from build123d import *

# Parameters (mm, degrees)
ESQUISSE1_W             = 27.85
ESQUISSE1_H             = 200
BOSS_EXTRU_1_DEPTH      = 6
ESQUISSE4_R             = 2.5
ENL_V_MAT_EXTRU_3_DEPTH = 29
ESQUISSE5_R             = 13.925
ENL_V_MAT_EXTRU_4_DEPTH = 3
ESQUISSE7_W             = 16.87
ESQUISSE7_H             = 23
ESQUISSE7_H_2           = 29
ENL_V_MAT_EXTRU_6_DEPTH = 13
CONG_1_R                = 10
CONG_2_R                = 10


with BuildPart() as part:
    # Esquisse1 → Boss.-Extru.1 (new body)
    with BuildSketch(Plane.XY):
        with Locations((4.111190476, -68.237738095)):
            Rectangle(ESQUISSE1_W, ESQUISSE1_H)
        with BuildLine():
            Line((-9.813809524, 31.762261905), (18.036190476, 31.762261905))
            ThreePointArc((18.036190476, 31.762261905), (4.111190476, 45.687261905), (-9.813809524, 31.762261905))
        make_face()
    extrude(amount=BOSS_EXTRU_1_DEPTH)

    # Esquisse4 → Enlèv. mat.-Extru.3 (cut)
    with BuildSketch(Plane.XY.offset(6)):
        with Locations((4.111190476, -160.237738095)):
            Circle(ESQUISSE4_R)
    extrude(amount=-ENL_V_MAT_EXTRU_3_DEPTH, mode=Mode.SUBTRACT)

    # Esquisse5 → Enlèv. mat.-Extru.4 (cut)
    with BuildSketch(Plane(origin=(0, 0, 0), x_dir=(-1, 0, 0), z_dir=(0, 0, -1))):
        with Locations((-4.111190476, 31.762261905)):
            Circle(ESQUISSE5_R)
    extrude(amount=-ENL_V_MAT_EXTRU_4_DEPTH, mode=Mode.SUBTRACT)

    # Esquisse7 → Enlèv. mat.-Extru.6 (cut)
    with BuildSketch(Plane(origin=(0, 0, 0), x_dir=(-1, 0, 0), z_dir=(0, 0, -1))):
        with BuildLine():
            ThreePointArc((-13.036190476, -115.237738095), (-4.601190476, -106.802738095), (3.833809524, -115.237738095))
            Line((3.833809524, -115.237738095), (-13.036190476, -115.237738095))
        make_face()
        with Locations((-4.601190476, -126.737738095)):
            Rectangle(ESQUISSE7_W, ESQUISSE7_H)
        with BuildLine():
            Line((-13.036190476, -138.237738095), (3.833809524, -138.237738095))
            ThreePointArc((3.833809524, -138.237738095), (-4.601190476, -146.672738095), (-13.036190476, -138.237738095))
        make_face()
        with BuildLine():
            Line((3.833809524, -93.237738095), (-13.036190476, -93.237738095))
            ThreePointArc((-13.036190476, -93.237738095), (-4.601190476, -101.672738095), (3.833809524, -93.237738095))
        make_face()
        with Locations((-4.601190476, -78.737738095)):
            Rectangle(ESQUISSE7_W, ESQUISSE7_H_2)
        with BuildLine():
            Line((3.833809524, -64.237738095), (-13.036190476, -64.237738095))
            ThreePointArc((-13.036190476, -64.237738095), (-4.601190476, -55.802738095), (3.833809524, -64.237738095))
        make_face()
        with BuildLine():
            ThreePointArc((3.833809524, -42.237738095), (-4.601190476, -50.672738095), (-13.036190476, -42.237738095))
            Line((-13.036190476, -42.237738095), (3.833809524, -42.237738095))
        make_face()
        with Locations((-4.601190476, -30.737738095)):
            Rectangle(ESQUISSE7_W, ESQUISSE7_H)
        with BuildLine():
            Line((3.833809524, -19.237738095), (-13.036190476, -19.237738095))
            ThreePointArc((-13.036190476, -19.237738095), (-4.601190476, -10.802738095), (3.833809524, -19.237738095))
        make_face()
    extrude(amount=-ENL_V_MAT_EXTRU_6_DEPTH, mode=Mode.SUBTRACT)

    # Congé1
    cong_1_edges = [part.edges().sort_by_distance(p)[0] for p in [
        (18.036190476, -168.237738095, 3),
    ]]
    fillet(cong_1_edges, radius=CONG_1_R)

    # Congé2
    cong_2_edges = [part.edges().sort_by_distance(p)[0] for p in [
        (-9.813809524, -168.237738095, 3),
    ]]
    fillet(cong_2_edges, radius=CONG_2_R)


solid = part.part
Here's how the part is built. I have some questions about the finished solid (model axes, mm). A direction names the side the tool comes from. Coordinates: 2 decimals unless noted, no trailing zeros. Loops run counter-clockwise (first coordinate to the right, second up) from the corner with the lowest first, then second, coordinate; pieces in that order, holes last. Notation, with made-up numbers: (60, 16.25) -> (87, 16.25) arc R15 ccw to (87, 23.25) -> close; hole circle Ø1 at (12, 54.5). An arc over 180 degrees is marked (long way). Use one line per item in the form item = value. Start each with the question number.
(1) On a 3-axis mill with a long thin cutter (end or side, diameter ignored), from which of +Z, -Z, +X, -X, +Y, -Y can I reach the whole of each face in a straight line? I mean faces 1 (the face through (-6.807, -165.386, 3.042)), 2 (the face through (4.787, -10.805, 2.958)), 3 (the face through (4, 32, 3)). Say none if no direction works.
(2) If we section it at B-B (z = 1.8): Please give me the cut outline in (x, y) (3 decimals), then the cut area to 3 significant figures.
(3) If we section it at A-A (y = -47): Please give me the cut outline in (x, z), then the cut area to 3 significant figures.
(4) If we section it at C-C (y = -142): Please give me the cut outline in (x, z).
(5) We'd pull the mould along X, two halves only. Please class faces 4 (the face through (18.036, -65, 3)), 5 (the face through (3.79, -157.76, 3.04)), 6 (the face through (-9.814, -65, 3)), 7 (the face through (-5, -60, 6)): pulls with the +X half, pulls with the -X half, needs draft (parallel to the pull), parting line crosses it, or undercut.
(6) Will these pins go through, and if not, where does the flat tip stop? pin 1 (3 mm diameter, centred on x = 12, z = 1, fed in from +Y); pin 2 (2 mm diameter, centred on x = 15, z = 5, fed in from +Y).
(7) Please list where these lines run through material, in increasing order: line 1 along Y through (x, z) = (12.25, 4.55); line 2 along X through (y, z) = (-21.5, 0.5); line 3 along Y through (x, z) = (11, 1.85).
Verdict:
q1.face_1 = +Z, -Z, -X, -Y
q1.face_2 = +Z, -Z
q1.face_3 = -Z, +Y
q2.outline = (-9.814, -158.238) arc R10 ccw to (0.186, -168.238) -> (8.036, -168.238) arc R10 ccw to (18.036, -158.238) -> (18.036, 31.762) arc R13.925 cw to (-9.814, 31.762) -> close; hole (-3.834, -138.238) arc R8.435 ccw to (13.036, -138.238) -> (13.036, -115.238) arc R8.435 ccw to (-3.834, -115.238) -> close; hole (-3.834, -93.238) arc R8.435 ccw to (13.036, -93.238) -> (13.036, -64.238) arc R8.435 ccw to (-3.834, -64.238) -> close; hole (-3.834, -42.238) arc R8.435 ccw to (13.036, -42.238) -> (13.036, -19.238) arc R8.435 ccw to (-3.834, -19.238) -> close; hole circle Ø5 at (4.111, -160.238)
q2.area = 3,270 mm²
q3.outline = (-9.81, 0) -> (-2.36, 0) -> (-2.36, 6) -> (-9.81, 6) -> close; (11.56, 0) -> (18.04, 0) -> (18.04, 6) -> (11.56, 6) -> close
q3.area = 83.6 mm²
q4.outline = (-9.81, 0) -> (-2.95, 0) -> (-2.95, 6) -> (-9.81, 6) -> close; (12.15, 0) -> (18.04, 0) -> (18.04, 6) -> (12.15, 6) -> close
q5.face_4 = pulls with the +X half
q5.face_5 = undercut
q5.face_6 = pulls with the -X half
q5.face_7 = needs draft
q6.pin_1 = 21.48
q6.pin_2 = 41.57
q7.line_1 = -167.31 to -141.79, -111.68 to -96.79, -60.68 to -45.79, -15.68 to 43.06
q7.line_2 = -9.81 to -3.83, 13.04 to 18.04
q7.line_3 = -167.79 to -143.73, -109.74 to -98.73, -58.74 to -47.73, -13.74 to 19.66
